Build history of the part. All positions in model axes, mm. Face numbers are marked on the shaded views. A direction names the side the tool comes from. Give positions to 0.01 mm unless a question says otherwise; leave off trailing zeros. Write each loop counter-clockwise with the first axis right and the second up, starting at its lowest first coordinate (ties: lowest second). Pieces come first, ordered by that corner, then holes. Notation, with made-up numbers: M 67,58.5 L 91,58.5 A13 ccw 91,69.5 Z; hole C 9.5,-2.5 d7. An arc over 180 degrees is marked long. One line per item, written item: value. Start each with the question number.
from build123d import *

# Parameters (mm, degrees)
SKETCH_1_R             = 2.5
EXTRUDE_1_DEPTH        = 20
SKETCH_2_W             = 10
SKETCH_2_H             = 20
EXTRUDE_2_DEPTH        = 3
SKETCH_3_R             = 1.75
CUT_EXTRUDE_1_DEPTH    = 4
FILLET_1_R             = 3
FILLET_1_OF_MIRROR_1_R = 3
CHAMFER_1_SIZE         = 1


with BuildPart() as part:
    # ｽｹｯﾁ1 → ﾎﾞｽ - 押し出し1 (new body, symmetric)
    with BuildSketch(Plane.XY):
        with BuildLine():
            Line((-5, 0), (5, 0))
            Line((5, 0), (5, 7))
            ThreePointArc((5, 7), (0, 12), (-5, 7))
            Line((-5, 7), (-5, 0))
        make_face()
        with Locations((0, 7)):
            Circle(SKETCH_1_R, mode=Mode.SUBTRACT)
    extrude(amount=EXTRUDE_1_DEPTH, both=True)

    # ｽｹｯﾁ2 → ﾎﾞｽ - 押し出し2 (add)
    with BuildSketch(Plane.XZ):
        with Locations((0, 20)):
            Rectangle(SKETCH_2_W, SKETCH_2_H)
    extrude_2 = extrude(amount=EXTRUDE_2_DEPTH)

    # ｽｹｯﾁ3 → ｶｯﾄ - 押し出し1 (cut, through all)
    with BuildSketch(Plane(origin=(0, 0, 0), x_dir=(1, 0, 0), z_dir=(0, 1, 0))):
        with Locations((0, -25)):
            Circle(SKETCH_3_R)
    cut_extrude_1 = extrude(amount=-CUT_EXTRUDE_1_DEPTH, mode=Mode.SUBTRACT)

    # ﾌｨﾚｯﾄ1
    fillet_1_edges = [part.edges().sort_by_distance(p)[0] for p in [
        (-5, -1.5, 30),
        (5, -1.5, 30),
    ]]
    fillet(fillet_1_edges, radius=FILLET_1_R)

    # ﾐﾗｰ1: ﾎﾞｽ - 押し出し2, ｶｯﾄ - 押し出し1 across plane
    add(extrude_2.mirror(Plane.XY))
    add(cut_extrude_1.mirror(Plane.XY), mode=Mode.SUBTRACT)

    # ﾌｨﾚｯﾄ1 of ﾐﾗｰ1
    fillet_1_of_mirror_1_edges = [part.edges().sort_by_distance(p)[0] for p in [
        (-5, -1.5, -30),
        (5, -1.5, -30),
    ]]
    fillet(fillet_1_of_mirror_1_edges, radius=FILLET_1_OF_MIRROR_1_R)

    # 面取り1
    chamfer_1_edges = [part.edges().sort_by_distance(p)[0] for p in [
        (-2.5, 7, -20),
        (-2.5, 7, 20),
    ]]
    chamfer(chamfer_1_edges, length=CHAMFER_1_SIZE)


solid = part.part
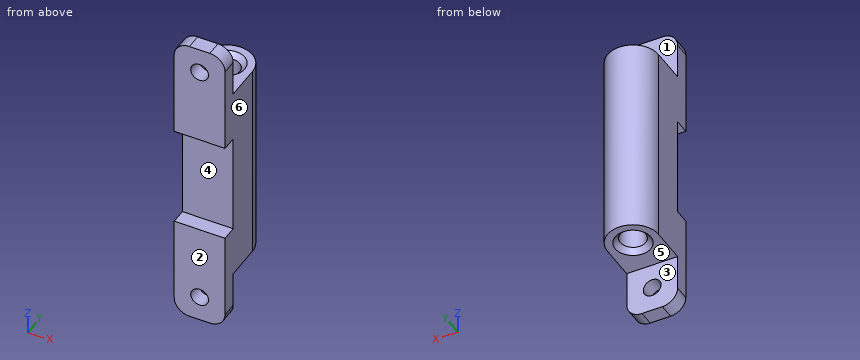
1) Tool access for the marked faces 1, 2 and 3: list every direction of +Z, -Z, +X, -X, +Y, -Y with a clear straight run to the whole face (end or side of a thin tool).
2) Band-saw the part on D-D (y = 2.75). List the corners of the cut face in (x, z), then the cut area to 3 significant figures.
3) Band-saw the part on A-A (x = 0). List the corners of the cut face in (y, z).
4) Band-saw the part on C-C (z = 9). List the corners of the cut face in (x, y).
5) Mould opens along Z. For the marked faces 4, 5 and 6 say: released by +Z, released by -Z, zero draft, split by the parting line, or undercut.
6) Band-saw the part on B-B (z = -25). List the corners of the cut face in (x, y), then the cut area to 3 significant figures.
7) Drop flat-ended pins along their axis: P1, Ø5, axis at x = 3, y = 6, coming from the -Z side; P2, Ø3, axis at x = 0, z = 25, coming from the -Y side; P3, Ø3, axis at x = -2.5, y = 9.5, coming from the +Z side; P4, Ø1, axis at y = 8, z = 20, coming from the -X side. Give the stop position or say it passes through.
8) Probe line 1 along Y through (x, z) = (0, 12); line 2 along X through (y, z) = (-1.45, -25); line 3 along Y through (x, z) = (0, 0). List the from-to ranges inside material, lowest first. Write a range as from..to.
Model answer:
1. face 1: +Z, +X, -X, +Y
1. face 2: +Z, -Z, +X, -X, -Y
1. face 3: -Z, +X, -X, +Y
2. outline: M -5,-20 L 5,-20 L 5,20 L -5,20 Z
2. area: 400 mm²
3. outline: M -3,-30 L 0,-30 L 0,-26.75 L -3,-26.75 Z; M -3,-23.25 L 0,-23.25 L 0,-20 L 3.5,-20 L 4.5,-19 L 4.5,19 L 3.5,20 L 0,20 L 0,23.25 L -3,23.25 L -3,10 L 0,10 L 0,-10 L -3,-10 Z; M -3,26.75 L 0,26.75 L 0,30 L -3,30 Z; M 9.5,-19 L 10.5,-20 L 12,-20 L 12,20 L 10.5,20 L 9.5,19 Z
4. outline: M -5,0 L 5,0 L 5,7 A5 ccw -5,7 Z; hole C 0,7 d5
5. face 4: undercut
5. face 5: released by -Z
5. face 6: zero draft
6. outline: M -5,-3 L -1.75,-3 L -1.75,0 L -5,0 Z; M 1.75,-3 L 5,-3 L 5,0 L 1.75,0 Z
6. area: 19.5 mm²
7. P1: stops at z = -20
7. P2: passes through
7. P3: stops at z = 20
7. P4: stops at x = -4.97
8. line 1: y = -3..4.5, 9.5..12
8. line 2: x = -5..-1.75, 1.75..5
8. line 3: y = 0..4.5, 9.5..12
